Autodesk Inventor part; units mm, degrees
ref_plane "YZ Plane" through (0, 0, 0) normal (1, 0, 0) x (0, 1, 0)
ref_plane "XZ Plane" through (0, 0, 0) normal (0, 1, 0) x (-1, 0, 0)
ref_plane "XY Plane" through (0, 0, 0) normal (0, 0, 1) x (1, 0, 0)
sketch "Sketch1" plane through (0, 0, 0) normal (0, 1, 0) x (-1, 0, 0)
  line L0 (-47.625, 80.645) -> (47.625, 80.645)
  line L1 (47.625, 80.645) -> (47.625, -80.645)
  line L2 (47.625, -80.645) -> (-47.625, -80.645)
  line L3 (-47.625, -80.645) -> (-47.625, 80.645)
  line L4 (-47.625, 80.645) -> (47.625, -80.645) construction
  line L5 (47.625, 80.645) -> (-47.625, -80.645) construction
  point P0 (0, 0)
  dimension "d0" = 161.29
  dimension "d1" = 95.25
extrude "Extrusion1" add sketch "Sketch1" along normal blind 6.35
sketch "Sketch3" plane through (0, 0, 0) normal (0, -1, 0) x (1, 0, 0)
  line L0 (-44.45, 77.47) -> (44.45, 77.47)
  line L1 (44.45, 77.47) -> (44.45, -77.47)
  line L2 (44.45, -77.47) -> (-44.45, -77.47)
  line L3 (-44.45, -77.47) -> (-44.45, 77.47)
  line L4 (-44.45, 77.47) -> (44.45, -77.47) construction
  line L5 (44.45, 77.47) -> (-44.45, -77.47) construction
  line L6 (-41.275, 74.295) -> (41.275, 74.295)
  line L7 (41.275, 74.295) -> (41.275, -74.295)
  line L8 (41.275, -74.295) -> (-41.275, -74.295)
  line L9 (-41.275, -74.295) -> (-41.275, 74.295)
  line L10 (-41.275, 74.295) -> (41.275, -74.295) construction
  line L11 (41.275, 74.295) -> (-41.275, -74.295) construction
  point P0 (0, 0)
  dimension "d4" = 154.94
  dimension "d5" = 88.9
  dimension "d6" = 148.59
  dimension "d7" = 82.55
extrude "Extrusion2" add sketch "Sketch3" along normal blind 4.7625
sketch "Sketch4" plane through (0, 6.35, 0) normal (0, 1, 0) x (1, 0, 0)
  line L0 (24.765, -53.975) -> (-24.765, -53.975) construction
  line L1 (-24.765, -53.975) -> (-24.765, 53.975) construction
  line L2 (-24.765, 53.975) -> (24.765, 53.975) construction
  line L3 (24.765, 53.975) -> (24.765, -53.975) construction
  line L4 (24.765, -53.975) -> (-24.765, 53.975) construction
  line L5 (-24.765, -53.975) -> (24.765, 53.975) construction
  circle A0 centre (-24.765, -53.975) radius 10.9982
  circle A1 centre (-24.765, 53.975) radius 10.9982
  circle A2 centre (-24.765, -22.225) radius 10.9982
  circle A3 centre (-24.765, 22.225) radius 10.9982
  line L6 (47.625, -80.645) -> (47.625, 80.645)
  point P0 (0, 0)
  dimension "d12" = 21.9964
  dimension "d13" = 21.9964
  dimension "d15" = 21.9964
  dimension "d17" = 31.75
  dimension "d18" = 21.9964
  dimension "d19" = 31.75
  dimension "d25" = 44.45
  dimension "d26" = 72.39
extrude "Extrusion3" cut sketch "Sketch4" against normal up to next
fillet "Fillet1" radius 3.175 12 edges at (47.625, 3.175, 80.645) (-47.625, 3.175, 80.645) (47.625, 3.175, -80.645) (-47.625, 3.175, -80.645) (44.45, -2.3813, -77.47) (44.45, -2.3813, 77.47) (-44.45, -2.3813, -77.47) (-41.275, -2.3813, 74.295) (-44.45, -2.3813, 77.47) (41.275, -2.3813, 74.295) (41.275, -2.3813, -74.295) (-41.275, -2.3813, -74.295)
sketch "Sketch5" plane through (44.45, 0, -80.645) normal (0, 0, -1) x (-1, 0, 0)
  line L0 (88.9, 6.35) -> (0, 6.35)
  line L1 (40.1232, 6.35) -> (46.4732, 6.35)
  line L2 (46.4732, 6.35) -> (46.4732, 2.8141)
  line L3 (46.4732, 2.8141) -> (40.1232, 2.8141)
  line L4 (40.1232, 2.8141) -> (40.1232, 6.35)
  point P0 (44.45, 0)
  dimension "d37" = 6.35
sketch "Sketch6" plane through (-47.625, 0, -77.47) normal (-1, 0, 0) x (0, 0, 1)
  line L0 (0, 6.35) -> (154.94, 6.35)
  line L1 (88.6968, 6.35) -> (88.6968, 0)
  line L2 (82.3468, 6.35) -> (88.6968, 6.35)
  line L3 (88.6968, 6.35) -> (88.6968, 3.175)
  line L4 (88.6968, 3.175) -> (82.3468, 3.175)
  line L5 (82.3468, 3.175) -> (82.3468, 6.35)
  point P0 (77.47, 0)
  dimension "d38" = 6.35
sketch "Sketch7" plane through (47.625, 0, 77.47) normal (1, 0, 0) x (0, 0, -1)
  line L0 (154.94, 6.35) -> (0, 6.35)
  line L1 (66.2432, 6.35) -> (66.2432, 0)
  line L2 (72.5932, 6.35) -> (66.2432, 6.35)
  line L3 (66.2432, 6.35) -> (66.2432, 3.175)
  line L4 (66.2432, 3.175) -> (72.5932, 3.175)
  line L5 (72.5932, 3.175) -> (72.5932, 6.35)
  point P0 (77.47, 0)
  dimension "d36" = 6.35
sketch "Sketch8" plane through (-44.45, 0, 80.645) normal (0, 0, 1) x (1, 0, 0)
  line L0 (0, 6.35) -> (88.9, 6.35)
  line L1 (51.344, 6.35) -> (44.994, 6.35)
  line L2 (44.994, 6.35) -> (44.994, 2.9455)
  line L3 (44.994, 2.9455) -> (51.344, 2.9455)
  line L4 (51.344, 2.9455) -> (51.344, 6.35)
  point P0 (44.45, 0)
  dimension "d39" = 6.35
extrude "Extrusion4" add sketch "Sketch8" along normal blind 25.4
extrude "Extrusion5" add sketch "Sketch5" along normal blind 25.4
extrude "Extrusion6" add sketch "Sketch6" along normal blind 25.4
extrude "Extrusion7" add sketch "Sketch7" along normal blind 25.4
properties part number "iceTubeClockTop"
The listing builds one solid part. Answer for the finished solid, in the listing's coordinates (mm). A direction names the side the tool comes from. Coordinates: 2 decimals unless noted, no trailing zeros. Write each loop counter-clockwise with the first axis right and the second up, starting at its lowest first coordinate (ties: lowest second). Pieces come first, ordered by that corner, then holes. Notation, with made-up numbers: M 58.25,46 L 110.25,46 A22 ccw 110.25,81 Z; hole C -39.5,-8 d1. An arc over 180 degrees is marked long. Use one line per item in the form item = value.
Item 1: For faces 4 (the face through (-1, -2, 74.295)), 5 (the face through (-60, 3.175, 8)), 6 (the face through (1, 2.814, -93)), determine the directions among +Z, -Z, +X, -X, +Y, -Y from which every point of the face is accessible in a straight line to the end or side of a thin tool.
Model answer:
face_4 = -Y
face_5 = +Z, -Z, -X, -Y
face_6 = -Z, +X, -X, -Y
Item 2: Find section B-B, the plane y = -2.25. Give the vertices of the cut face in (x, z) (3 decimals), plus the area to 3 significant figures.
Model answer:
outline = M -44.45,-74.295 A3.175 ccw -41.275,-77.47 L 41.275,-77.47 A3.175 ccw 44.45,-74.295 L 44.45,74.295 A3.175 ccw 41.275,77.47 L -41.275,77.47 A3.175 ccw -44.45,74.295 Z; hole M -41.275,-71.12 A3.175 ccw -38.1,-74.295 L 38.1,-74.295 A3.175 ccw 41.275,-71.12 L 41.275,71.12 A3.175 ccw 38.1,74.295 L -38.1,74.295 A3.175 ccw -41.275,71.12 Z
area = 1,510 mm2
Item 3: Given P1, Ø1, axis at x = 59.5, y = 4, coming from the +Z side; P2, Ø1.9, axis at y = 3, z = -37.5, coming from the -X side (3 decimals); P3, Ø5, axis at x = -0.5, z = -97, coming from the -Y side, each flat-ended and moving along its own axis, determine where each tip first touches the part or whether it passes through.
Model answer:
P1 = 11.23
P2 = -47.625
P3 = 2.81
Item 4: Find section D-D, the plane x = -22. Give the number of separate pieces and of enclosed holes in the cut face, plus the area to 3 significant figures.
Model answer:
separate_pieces = 5
enclosed_holes = 0
area = 514 mm2
Item 5: The mould has two halves that part along X. Classify faces 1 (the face through (-43, -4.762, 23)), 2 (the face through (-41.275, -2, -1)), 3 (the face through (-44.45, -2, -1)): released by +X, released by -X, zero draft, split by the parting line, or undercut.
Model answer:
face_1 = zero draft
face_2 = undercut
face_3 = released by -X
Item 6: Find the intervals of material crossed by probe 1 along Z at (x, y) = (-25.5, 5.25) (3 decimals); probe 2 along X at (y, z) = (-1, 23.5) (3 decimals); probe 3 along Z at (x, y) = (-18, -3) (3 decimals), in increasing order.
Model answer:
probe_1 = -80.645 to -64.949, -43.001 to -33.199, -11.251 to 11.251, 33.199 to 43.001, 64.949 to 80.645
probe_2 = -44.45 to -41.275, 41.275 to 44.45
probe_3 = -77.47 to -74.295, 74.295 to 77.47
